Could you check a few things on this model? Use its own coordinates, in mm. A direction names the side the tool comes from. Coordinates: 2 decimals unless noted, no trailing zeros. Order: outer loops, then holes, each group sorted by start corner. A loop starts at its lowest first (then second) coordinate and runs counter-clockwise, first axis right, second up. Notation, with made-up numbers: (35, 28.25) - (84, 28.25) arc R34 cw to (84, 60.25) - close; hole circle Ø10 at (-21, 68). An arc over 180 degrees is marked (long way). One line per item, written item: value.
from build123d import *

# Parameters (mm, degrees)
SKETCH_1_R                = 4.5
EXTRUDE_1_DEPTH           = 5
SKETCH_2_R                = 3.65
EXTRUDE_2_DEPTH           = 10
SKETCH_3_R                = 4.5
EXTRUDE_3_DEPTH           = 5
CHAMFER_2_SIZE            = 1
CHAMFER_3_SIZE            = 1
HOLE_WIZARD_5_0_5_1_D     = 5
HOLE_WIZARD_5_0_5_1_DEPTH = 5
HOLE_WIZARD_5_0_5_1_TIP   = 1.502151548
HOLE_WIZARD_3_0_3_1_D     = 3
HOLE_WIZARD_3_0_3_1_DEPTH = 5
HOLE_WIZARD_3_0_3_1_TIP   = 0.901290929
M3X0_5_1_REACH            = 24.389
M3X0_5_1_BORE_R           = 1.25


with BuildPart() as part:
    # 草圖1 → 填料-伸長1 (new body)
    with BuildSketch(Plane.XY):
        Circle(SKETCH_1_R)
    extrude(amount=EXTRUDE_1_DEPTH)

    # 草圖2 → 填料-伸長2 (add)
    with BuildSketch(Plane.XY.offset(5)):
        Circle(SKETCH_2_R)
    extrude(amount=EXTRUDE_2_DEPTH)

    # 草圖3 → 填料-伸長3 (add)
    with BuildSketch(Plane.XY.offset(15)):
        Circle(SKETCH_3_R)
    extrude(amount=EXTRUDE_3_DEPTH)

    # 導角2
    # the kernel refuses this chamfer: 1 mm, written as the material it adds along each edge
    with BuildSketch(Plane(origin=(0, 0, 5), x_dir=(1, 0, 0), z_dir=(0, -1, 0))) as chamfer_2_piece_1_section:
        Polygon((3.65, CHAMFER_2_SIZE), (3.65 + CHAMFER_2_SIZE, 0), (3.65, 0), align=None)
    chamfer_2_piece_1 = revolve(axis=Axis((0, 0, 5), (0, 0, 1)), mode=Mode.PRIVATE)
    chamfer_2_piece_1 = chamfer_2_piece_1 & Plane(origin=(0, 0, 5.572415942), x_dir=(1, 0, 0), z_dir=(0, 0, -1)) * Cylinder(4.5, 19, mode=Mode.PRIVATE)
    add(chamfer_2_piece_1)

    # 導角3
    # the kernel refuses this chamfer: 1 mm, written as the material it adds along each edge
    with BuildSketch(Plane(origin=(0, 0, 15), x_dir=(1, 0, 0), z_dir=(0, -1, 0))) as chamfer_3_piece_1_section:
        Polygon((3.65, -CHAMFER_3_SIZE), (3.65 + CHAMFER_3_SIZE, 0), (3.65, 0), align=None)
    chamfer_3_piece_1 = revolve(axis=Axis((0, 0, 15), (0, 0, 1)), mode=Mode.PRIVATE)
    chamfer_3_piece_1 = chamfer_3_piece_1 & Plane(origin=(0, 0, 14.427584058), x_dir=(1, 0, 0), z_dir=(0, 0, -1)) * Cylinder(4.5, 19, mode=Mode.PRIVATE)
    add(chamfer_3_piece_1)

    # Ø5.0 (5) 直徑孔1
    with Locations(Plane.XY.offset(20)):
        with Locations((0, 0)):
            Hole(HOLE_WIZARD_5_0_5_1_D / 2, depth=HOLE_WIZARD_5_0_5_1_DEPTH)
            with Locations((0, 0, -(HOLE_WIZARD_5_0_5_1_DEPTH + HOLE_WIZARD_5_0_5_1_TIP / 2))):  # 118° drill point
                Cone(0, HOLE_WIZARD_5_0_5_1_D / 2, HOLE_WIZARD_5_0_5_1_TIP, mode=Mode.SUBTRACT)

    # Ø3.0 (3) 直徑孔1
    with Locations(Plane(origin=(0, 0, 0), x_dir=(-1, 0, 0), z_dir=(0, 0, -1))):
        with Locations((0, 0)):
            Hole(HOLE_WIZARD_3_0_3_1_D / 2, depth=HOLE_WIZARD_3_0_3_1_DEPTH)
            with Locations((0, 0, -(HOLE_WIZARD_3_0_3_1_DEPTH + HOLE_WIZARD_3_0_3_1_TIP / 2))):  # 118° drill point
                Cone(0, HOLE_WIZARD_3_0_3_1_D / 2, HOLE_WIZARD_3_0_3_1_TIP, mode=Mode.SUBTRACT)

    # M3x0.5  螺絲攻的螺孔鑽1 bore → M3x0.5  螺絲攻的螺孔鑽1 (cut, up to next)
    with BuildSketch(Plane(origin=(0, 4.5, 0), x_dir=(1, 0, 0), z_dir=(0, 1, 0)), mode=Mode.PRIVATE) as m3x0_5_1_sk1:
        with Locations((0, -2.5)):
            Circle(M3X0_5_1_BORE_R)
    m3x0_5_1_tool1 = extrude(m3x0_5_1_sk1.sketch, amount=-M3X0_5_1_REACH, mode=Mode.PRIVATE) & part.part
    m3x0_5_1 = m3x0_5_1_tool1.solids().sort_by_distance((0, 4.5, 2.5))[0]
    add(m3x0_5_1, mode=Mode.SUBTRACT)

    # 鏡射1: M3x0.5  螺絲攻的螺孔鑽1 across plane
    add(m3x0_5_1.mirror(Plane(origin=(0, 0, 10), x_dir=(1, 0, 0), z_dir=(0, 0, -1))), mode=Mode.SUBTRACT)


solid = part.part
Item 1: I want a section at D-D on z = 2.5. Please give me the cut outline in (x, y), then the cut area to 3 significant figures.
Conclusion:
outline: (-1.25, 0.83) - (-1.25, 4.32) arc R4.5 ccw (long way) to (1.25, 4.32) - (1.25, 0.83) arc R1.5 cw (long way) to start
area: 48.7 mm²
Item 2: I want a section at C-C on z = 18. Please give me the cut outline in (x, y), then the cut area to 3 significant figures.
Conclusion:
outline: (-1.15, 2.22) - (-1.15, 4.35) arc R4.5 ccw (long way) to (1.15, 4.35) - (1.15, 2.22) arc R2.5 cw (long way) to start
area: 39.3 mm²
Item 3: I want a section at A-A on z = 7.25. Please give me the cut outline in (x, y), then the cut area to 3 significant figures.
Conclusion:
outline: circle Ø7.3 at (0, 0)
area: 41.9 mm²
Item 4: For faces 1 (the face through (-0.99, 3.35, 16.74)), 2 (the face through (3.48, 1.1, 9.94)), 3 (the face through (-0.325, -1.464, 2.535)), which set-ups out of +Z, -Z, +X, -X, +Y, -Y let a thin tool reach every point of the face, with its end or its side?
Conclusion:
face 1: +Y
face 2: none
face 3: -Z
Item 5: If I drill on probe 1 along Z at (x, y) = (0, 2.7); probe 2 along X at (y, z) = (0, 1.5); probe 3 along X at (y, z) = (0, 18.85), over which ranges is the centre line in solid material (lowest first)?
Conclusion:
probe 1: 0 to 1.25, 3.75 to 16.25, 18.75 to 20
probe 2: -4.5 to -1.5, 1.5 to 4.5
probe 3: -4.5 to -2.5, 2.5 to 4.5
Item 6: I want a section at B-B on x = -1. Give the number of separate pieces and of enclosed holes in the cut face, then the cut area to 3 significant figures.
Conclusion:
separate pieces: 3
enclosed holes: 0
area: 115 mm²
Item 7: Thinking about a two-plate mould opening in X: for faces 4 (the face through (0.54, -2.44, 17.46)), 5 (the face through (2, -2, 20)), 6 (the face through (-0.59, -4.46, 17.39)), which applies, pulls with the +X half, pulls with the -X half, needs draft (parallel to the pull), parting line crosses it, or undercut?
Conclusion:
face 4: undercut
face 5: needs draft
face 6: parting line crosses it
Item 8: I'm going to push flat-ended pins straight in: pin 1 Ø2.5 at (x, y) = (0, 0) entering from -Z; pin 2 Ø3 at (y, z) = (2.5, 13) entering from +X; pin 3 Ø1 at (x, z) = (-1.5, 14) entering from -Y. Where does each tip first touch, or does it pass through?
Conclusion:
pin 1: z = 5.15
pin 2: x = 3.55
pin 3: y = -3.9
